```python
from build123d import *

# Parameters (mm, degrees)
F1_DEPTH = 550
F2_R     = 2.2
F3_DEPTH = 1


with BuildPart() as f1:
    # F0 (on Front) → F1 (new body)
    with BuildSketch(Plane.XZ):
        Polygon((5, 13), (5, 12), (13, 12), (13, 33.2), (5, 33.2), (5, 32.2), (6, 32.2), (12, 32.2), (12, 13), (6, 13), align=None)
    extrude(amount=-F1_DEPTH)

    # F2 (on face) → F3 (cut)
    with BuildSketch(Plane.YZ.offset(13)):
        with Locations((26, 22.6)):
            Circle(F2_R)
        with Locations((128, 22.6)):
            Circle(F2_R)
        with Locations((416, 22.6)):
            Circle(F2_R)
        with Locations((492, 22.6)):
            Circle(F2_R)
    extrude(amount=-F3_DEPTH, mode=Mode.SUBTRACT)


solid = f1.part
```
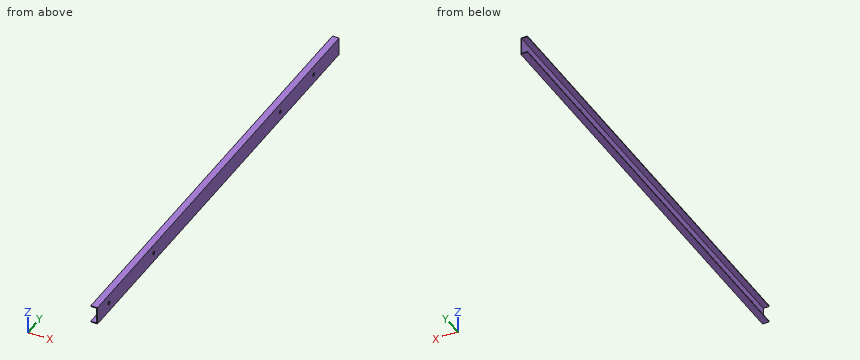
Input: part model. Units: mm. Frame: model coordinates. Give positions to 0.01 mm unless a question says otherwise; leave off trailing zeros. Write each loop counter-clockwise with the first axis right and the second up, starting at its lowest first coordinate (ties: lowest second). Pieces come first, ordered by that corner, then holes. Notation, with made-up numbers: (-19, 58.25) - (-3, 58.25) arc R22 ccw to (-3, 77.25) - close; hole circle Ø11 at (61, -27). An arc over 180 degrees is marked (long way). Write item = value, one per line. Start each with the question number.
1) Cut plane B-B (y = 438.5). Return loops of the section in (x, z).
2) Cut plane A-A (x = 6.75). Return loops of the section in (y, z).
3) Pin query (flat end, axial travel): pin 1 (1 mm diameter, centred on y = 372.5, z = 20, fed in from -X); pin 2 (3.5 mm diameter, centred on y = 128, z = 22.6, fed in from +X). Return the tip coordinate at first contact, or that it passes through.
4) Material intervals for L1, parallel to Z at x = 12.6, y = 416; L2, parallel to Z at x = 9.25, y = 245; L3, parallel to X at y = 173.5, z = 16, sorted ascending. Write a range as [from, to].
Answers follow:
q1.outline = (5, 12) - (13, 12) - (13, 33.2) - (5, 33.2) - (5, 32.2) - (12, 32.2) - (12, 13) - (5, 13) - close
q2.outline = (0, 12) - (550, 12) - (550, 13) - (0, 13) - close; (0, 32.2) - (550, 32.2) - (550, 33.2) - (0, 33.2) - close
q3.pin_1 = 12
q3.pin_2 = through
q4.L1 = [12, 20.4], [24.8, 33.2]
q4.L2 = [12, 13], [32.2, 33.2]
q4.L3 = [12, 13]
